Work out the finished part from the listing and answer in its coordinate system (mm). A direction names the side the tool comes from. Coordinates: 2 decimals unless noted, no trailing zeros. Order: outer loops, then holes, each group sorted by start corner. A loop starts at its lowest first (then second) coordinate and runs counter-clockwise, first axis right, second up.
1. The part is cut by section B-B, the plane z = -149. Give the vertices of the cut face in (x, y).
2. A tool of negligible diameter and unlimited length cuts with its end or side. For faces 4 (the flat face through (39.526, 14, -6)), 5 (the flat face through (46, 14, -12.7)), 6 (the flat face through (-189.074, 77, -104)), from which of +Z, -Z, +X, -X, +Y, -Y can it reach the whole face along a straight path? Write none if from no direction.
3. Flat-ended cylindrical pins translate along their axes: pin 1 Ø10 at (x, z) = (47.5, -42.5) entering from -Y; pin 2 Ø6 at (x, y) = (4.5, 108) entering from -Z. Find the tip coordinate at first contact, or state that the pin passes through.
4. The part is cut by section C-C, the plane x = -25.5. Give the vertices of the cut face in (y, z).
5. The part is cut by section D-D, the plane z = -41.5. Give the vertices of the cut face in (x, y), then the cut area to 3 significant figures.
6. The part is cut by section A-A, the plane y = 37. Give the vertices of the cut face in (x, z), then the cut area to 3 significant figures.
7. Determine the mould class of faces 1 (the flat face through (52.226, 77, -98)), 2 (the flat face through (46, 14, -88.9)), 3 (the flat face through (-102, 106, -12.7)) for opening direction X: +X half, -X half, draft (parallel to the pull), parting line (faces both ways), or undercut.
8. Find the intervals of material crossed by probe 1 along Y at (x, z) = (-98.5, -150); probe 2 along X at (y, z) = (190.5, -53); probe 3 along Z at (x, y) = (-166.5, -31.5), in increasing order.
```python
from build123d import *

# Parameters (mm, degrees)
F0_W          = 254
F0_H          = 254
F0_W_2        = 228.6
F0_H_2        = 228.6
F1_DEPTH      = 203.2
F2_T          = -12.7
F3_W          = 152.4
F3_H          = 101.6
F4_DEPTH      = 12.7
F5_W          = 101.6
F5_H          = 76.2
F6_DEPTH      = 76.2
F7_R          = 5.08
F8_R          = 5.08
F9_T1_DEPTH   = 269.24
F10_T1_DEPTH  = 269.24
F10_T3_DEPTH  = 228.6
F10_T5_DEPTH  = 228.6
F10_T11_DEPTH = 241.3
F10_T15_DEPTH = 241.3
F10_T22_DEPTH = 241.3
F10_T26_DEPTH = 241.3
F10_T33_DEPTH = 241.3
F10_T37_DEPTH = 241.3
F10_T44_DEPTH = 241.3
F10_T48_DEPTH = 241.3


# Not quite as in the source:
# - a fillet or chamfer that OpenCascade refuses, or shapes differently, is made with other operations: its cross-section is extruded or revolved along the edge and cut away or added


with BuildPart() as f1:
    # F0 (on Top) → F1 (new body)
    with BuildSketch(Plane.XY):
        with Locations((-74.773899883, 78.5929929912)):
            Rectangle(F0_W, F0_H)
        with Locations((-74.773899883, 78.5929929912)):
            Rectangle(F0_W_2, F0_H_2, mode=Mode.SUBTRACT)
        with Locations((-74.773899883, 78.5929929912)):
            Rectangle(F0_W_2, F0_H_2)
    extrude(amount=-F1_DEPTH)

    # F2
    f2_openings = [f1.faces().sort_by_distance(p)[0] for p in [
        (-74.7739, 78.592993, -203.2),
    ]]
    offset(amount=F2_T, openings=f2_openings)

    # F3 (on Top) → F4 (cut)
    with BuildSketch(Plane.XY):
        with Locations((-36.673899883, 15.0929929912)):
            Rectangle(F3_W, F3_H)
    extrude(amount=-F4_DEPTH, mode=Mode.SUBTRACT)

    # F5 (on Right) → F6 (cut)
    with BuildSketch(Plane.YZ):
        with Locations((15.0929929912, -50.8)):
            Rectangle(F5_W, F5_H)
    extrude(amount=F6_DEPTH, mode=Mode.SUBTRACT)

    # F7
    f7_edges = [f1.edges().sort_by_distance(p)[0] for p in [
        (52.2261, 205.592993, -101.6),
        (-201.7739, 205.592993, -101.6),
        (-74.7739, 205.592993, 0),
        (-74.7739, 205.592993, -203.2),
    ]]
    fillet(f7_edges, radius=F7_R)

    # F8
    f8_edges = [f1.edges().sort_by_distance(p)[0] for p in [
        (-201.7739, -48.407007, -101.6),
        (52.2261, -48.407007, -101.6),
        (-74.7739, -48.407007, 0),
        (-74.7739, -48.407007, -203.2),
    ]]
    fillet(f8_edges, radius=F8_R)

    # F9: fillet of radius 5.08 on 4 edges, made by hand

    # F9_s2 → F9_t1 (cut)
    with BuildSketch(Plane.XZ.offset(-213.2129929912)):
        with BuildLine():
            ThreePointArc((-196.693899883, 0), (-200.2860023315, -1.4878975516), (-201.773899883, -5.08))
            Line((-201.773899883, -5.08), (-201.773899883, 0))
            Line((-201.773899883, 0), (-196.693899883, 0))
        make_face()
        with BuildLine():
            ThreePointArc((-196.693899883, -203.2), (-200.2860023315, -201.7121024484), (-201.773899883, -198.12))
            Line((-201.773899883, -198.12), (-201.773899883, -203.2))
            Line((-201.773899883, -203.2), (-196.693899883, -203.2))
        make_face()
    extrude(amount=F9_T1_DEPTH, mode=Mode.SUBTRACT)

    # F10: fillet of radius 5.08 on 8 edges, made by hand

    # F10_s2 → F10_t1 (cut)
    with BuildSketch(Plane.XZ.offset(-213.2129929912)):
        with BuildLine():
            ThreePointArc((52.226100117, -198.12), (50.7382025654, -201.7121024484), (47.146100117, -203.2))
            Line((47.146100117, -203.2), (52.226100117, -203.2))
            Line((52.226100117, -203.2), (52.226100117, -198.12))
        make_face()
    extrude(amount=F10_T1_DEPTH, mode=Mode.SUBTRACT)

    # F10_s4 → F10_t3 (cut)
    with BuildSketch(Plane.XZ.offset(-192.8929929912)):
        with BuildLine():
            ThreePointArc((44.606100117, -203.2), (41.0139976685, -201.7121024484), (39.526100117, -198.12))
            Line((39.526100117, -198.12), (39.526100117, -203.2))
            Line((39.526100117, -203.2), (44.606100117, -203.2))
        make_face()
        with BuildLine():
            ThreePointArc((-194.153899883, -203.2), (-190.5617974346, -201.7121024484), (-189.073899883, -198.12))
            Line((-189.073899883, -198.12), (-189.073899883, -203.2))
            Line((-189.073899883, -203.2), (-194.153899883, -203.2))
        make_face()
    extrude(amount=F10_T3_DEPTH, mode=Mode.SUBTRACT)

    # F10_s6 → F10_t5 (cut)
    with BuildSketch(Plane.YZ.offset(-189.073899883)):
        with BuildLine():
            ThreePointArc((-40.7870070088, -203.2), (-37.1949045604, -201.7121024484), (-35.7070070088, -198.12))
            Line((-35.7070070088, -198.12), (-35.7070070088, -203.2))
            Line((-35.7070070088, -203.2), (-40.7870070088, -203.2))
        make_face()
        with BuildLine():
            ThreePointArc((197.9729929912, -203.2), (194.3808905428, -201.7121024484), (192.8929929912, -198.12))
            Line((192.8929929912, -198.12), (192.8929929912, -203.2))
            Line((192.8929929912, -203.2), (197.9729929912, -203.2))
        make_face()
    extrude(amount=F10_T5_DEPTH, mode=Mode.SUBTRACT)


with BuildPart() as f10_tool9:
    # F10_s10 → F10_t11 (new body)
    with BuildSketch(Plane.XZ.offset(48.4070070088)):
        with BuildLine():
            ThreePointArc((44.606100117, -203.2), (41.0139976685, -201.7121024484), (39.526100117, -198.12))
            Line((39.526100117, -198.12), (39.526100117, -203.2))
            Line((39.526100117, -203.2), (44.606100117, -203.2))
        make_face()
    extrude(amount=-F10_T11_DEPTH)

    split(bisect_by=Plane.XZ.offset(35.7070070088), keep=Keep.TOP)


with BuildPart() as f10_tool13:
    # F10_s14 → F10_t15 (new body)
    with BuildSketch(Plane.YZ.offset(-189.073899883)):
        with BuildLine():
            ThreePointArc((-40.7870070088, -203.2), (-37.1949045604, -201.7121024484), (-35.7070070088, -198.12))
            Line((-35.7070070088, -198.12), (-35.7070070088, -203.2))
            Line((-35.7070070088, -203.2), (-40.7870070088, -203.2))
        make_face()
    extrude(amount=F10_T15_DEPTH)

    split(bisect_by=Plane.YZ.offset(39.526100117), keep=Keep.TOP)


with BuildPart() as f10_tool9_1:
    add(f10_tool9.part)

    # F10_t17: intersect F10_tool13
    add(f10_tool13.part, mode=Mode.INTERSECT)


with BuildPart() as f1_1:
    add(f1.part)

    # F10_t7: cut F10_tool9
    add(f10_tool9_1.part, mode=Mode.SUBTRACT)


with BuildPart() as f10_tool20:
    # F10_s21 → F10_t22 (new body)
    with BuildSketch(Plane.XZ.offset(35.7070070088)):
        with BuildLine():
            ThreePointArc((44.606100117, -203.2), (41.0139976685, -201.7121024484), (39.526100117, -198.12))
            Line((39.526100117, -198.12), (39.526100117, -203.2))
            Line((39.526100117, -203.2), (44.606100117, -203.2))
        make_face()
    extrude(amount=-F10_T22_DEPTH)

    split(bisect_by=Plane.XZ.offset(-192.8929929912), keep=Keep.BOTTOM)


with BuildPart() as f10_tool24:
    # F10_s25 → F10_t26 (new body)
    with BuildSketch(Plane.YZ.offset(52.226100117)):
        with BuildLine():
            ThreePointArc((197.9729929912, -203.2), (194.3808905428, -201.7121024484), (192.8929929912, -198.12))
            Line((192.8929929912, -198.12), (192.8929929912, -203.2))
            Line((192.8929929912, -203.2), (197.9729929912, -203.2))
        make_face()
    extrude(amount=-F10_T26_DEPTH)

    split(bisect_by=Plane.YZ.offset(39.526100117), keep=Keep.TOP)


with BuildPart() as f10_tool20_1:
    add(f10_tool20.part)

    # F10_t28: intersect F10_tool24
    add(f10_tool24.part, mode=Mode.INTERSECT)


with BuildPart() as f1_2:
    add(f1_1.part)

    # F10_t18: cut F10_tool20
    add(f10_tool20_1.part, mode=Mode.SUBTRACT)


with BuildPart() as f10_tool31:
    # F10_s32 → F10_t33 (new body)
    with BuildSketch(Plane.YZ.offset(-201.773899883)):
        with BuildLine():
            ThreePointArc((-40.7870070088, -203.2), (-37.1949045604, -201.7121024484), (-35.7070070088, -198.12))
            Line((-35.7070070088, -198.12), (-35.7070070088, -203.2))
            Line((-35.7070070088, -203.2), (-40.7870070088, -203.2))
        make_face()
    extrude(amount=F10_T33_DEPTH)

    split(bisect_by=Plane.YZ.offset(-189.073899883), keep=Keep.BOTTOM)


with BuildPart() as f10_tool35:
    # F10_s36 → F10_t37 (new body)
    with BuildSketch(Plane.XZ.offset(-192.8929929912)):
        with BuildLine():
            ThreePointArc((-194.153899883, -203.2), (-190.5617974346, -201.7121024484), (-189.073899883, -198.12))
            Line((-189.073899883, -198.12), (-189.073899883, -203.2))
            Line((-189.073899883, -203.2), (-194.153899883, -203.2))
        make_face()
    extrude(amount=F10_T37_DEPTH)

    split(bisect_by=Plane.XZ.offset(35.7070070088), keep=Keep.TOP)


with BuildPart() as f10_tool31_1:
    add(f10_tool31.part)

    # F10_t39: intersect F10_tool35
    add(f10_tool35.part, mode=Mode.INTERSECT)


with BuildPart() as f1_3:
    add(f1_2.part)

    # F10_t29: cut F10_tool31
    add(f10_tool31_1.part, mode=Mode.SUBTRACT)


with BuildPart() as f10_tool42:
    # F10_s43 → F10_t44 (new body)
    with BuildSketch(Plane.YZ.offset(39.526100117)):
        with BuildLine():
            ThreePointArc((197.9729929912, -203.2), (194.3808905428, -201.7121024484), (192.8929929912, -198.12))
            Line((192.8929929912, -198.12), (192.8929929912, -203.2))
            Line((192.8929929912, -203.2), (197.9729929912, -203.2))
        make_face()
    extrude(amount=-F10_T44_DEPTH)

    split(bisect_by=Plane.YZ.offset(-189.073899883), keep=Keep.BOTTOM)


with BuildPart() as f10_tool46:
    # F10_s47 → F10_t48 (new body)
    with BuildSketch(Plane.XZ.offset(-205.5929929912)):
        with BuildLine():
            ThreePointArc((-194.153899883, -203.2), (-190.5617974346, -201.7121024484), (-189.073899883, -198.12))
            Line((-189.073899883, -198.12), (-189.073899883, -203.2))
            Line((-189.073899883, -203.2), (-194.153899883, -203.2))
        make_face()
    extrude(amount=F10_T48_DEPTH)

    split(bisect_by=Plane.XZ.offset(-192.8929929912), keep=Keep.BOTTOM)


with BuildPart() as f10_tool42_1:
    add(f10_tool42.part)

    # F10_t50: intersect F10_tool46
    add(f10_tool46.part, mode=Mode.INTERSECT)


with BuildPart() as f1_4:
    add(f1_3.part)

    # F10_t40: cut F10_tool42
    add(f10_tool42_1.part, mode=Mode.SUBTRACT)


solid = f1_4.part
```
Geometry says:
1. outline: (-201.77, -43.33) arc R5.08 ccw to (-196.69, -48.41) - (47.15, -48.41) arc R5.08 ccw to (52.23, -43.33) - (52.23, 200.51) arc R5.08 ccw to (47.15, 205.59) - (-196.69, 205.59) arc R5.08 ccw to (-201.77, 200.51) - close; hole (-189.07, -35.71) - (39.53, -35.71) - (39.53, 192.89) - (-189.07, 192.89) - close
2. face 4: +Z, -Z
2. face 5: +X
2. face 6: -Z
3. pin 1: stops at y = -48.41
3. pin 2: stops at z = -12.7
4. outline: (-48.41, -198.12) arc R5.08 ccw to (-43.33, -203.2) - (-40.79, -203.2) arc R5.08 ccw to (-35.71, -198.12) - (-35.71, 0) - (-43.33, 0) arc R5.08 ccw to (-48.41, -5.08) - close; (65.89, -12.7) - (192.89, -12.7) - (192.89, -198.12) arc R5.08 ccw to (197.97, -203.2) - (200.51, -203.2) arc R5.08 ccw to (205.59, -198.12) - (205.59, -5.08) arc R5.08 ccw to (200.51, 0) - (65.89, 0) - close
5. outline: (-201.77, -43.33) arc R5.08 ccw to (-196.69, -48.41) - (47.15, -48.41) arc R5.08 ccw to (52.23, -43.33) - (52.23, -35.71) - (-189.07, -35.71) - (-189.07, 192.89) - (39.53, 192.89) - (39.53, 65.89) - (52.23, 65.89) - (52.23, 200.51) arc R5.08 ccw to (47.15, 205.59) - (-196.69, 205.59) arc R5.08 ccw to (-201.77, 200.51) - close
5. area: 10,900 mm2
6. outline: (-201.77, -198.12) arc R5.08 ccw to (-196.69, -203.2) - (-194.15, -203.2) arc R5.08 ccw to (-189.07, -198.12) - (-189.07, -12.7) - (-112.87, -12.7) - (-112.87, 0) - (-196.69, 0) arc R5.08 ccw to (-201.77, -5.08) - close; (39.53, -198.12) arc R5.08 ccw to (44.61, -203.2) - (47.15, -203.2) arc R5.08 ccw to (52.23, -198.12) - (52.23, -88.9) - (39.53, -88.9) - close; (39.53, -12.7) - (52.23, -12.7) - (52.23, 0) - (39.53, 0) - close
6. area: 5,130 mm2
7. face 1: +X half
7. face 2: draft
7. face 3: undercut
8. probe 1: y = -48.41 to -35.71, 192.89 to 205.59
8. probe 2: x = -201.77 to -189.07, 39.53 to 52.23
8. probe 3: z = -12.7 to 0
